from build123d import *

# Parameters (mm, degrees)
F1_DEPTH = 10
F2_R     = 4


with BuildPart() as f1:
    # F0 (on Top) → F1 (new body)
    with BuildSketch(Plane.XY):
        with BuildLine():
            Line((-14.4176203235, -8.0238534513), (-15.1564685919, -6.5216148171))
            ThreePointArc((-15.1564685919, -6.5216148171), (-14.8061090102, -7.2821106815), (-14.4176203235, -8.0238534513))
        make_face()
        with BuildLine():
            ThreePointArc((14.4176203235, -8.0238534513), (0, -16.5), (-14.4176203235, -8.0238534513))
            Line((-14.4176203235, -8.0238534513), (0, -37.3379997909))
            Line((0, -37.3379997909), (14.4176203235, -8.0238534513))
        make_face()
        with BuildLine():
            ThreePointArc((14.4176203235, -8.0238534513), (14.8061090102, -7.2821106815), (15.1564685919, -6.5216148171))
            Line((15.1564685919, -6.5216148171), (14.4176203235, -8.0238534513))
        make_face()
        with BuildLine():
            ThreePointArc((15.1564685919, -6.5216148171), (16.1606270263, -3.329284325), (16.5, 0))
            ThreePointArc((16.5, 0), (-3.329284325, 16.1606270263), (-15.1564685919, -6.5216148171))
            Line((-15.1564685919, -6.5216148171), (-14.4176203235, -8.0238534513))
            ThreePointArc((-14.4176203235, -8.0238534513), (0, -16.5), (14.4176203235, -8.0238534513))
            Line((14.4176203235, -8.0238534513), (15.1564685919, -6.5216148171))
        make_face()
    extrude(amount=F1_DEPTH)

    # F2
    f2_edges = [f1.edges().sort_by_distance(p)[0] for p in [
        (0, -37.338, 5),
    ]]
    fillet(f2_edges, radius=F2_R)


solid = f1.part
Geometry check sheet. Reference: the model listing, model coordinates, mm. Give positions to 0.01 mm unless a question says otherwise; leave off trailing zeros. Order: outer loops, then holes, each group sorted by start corner. A loop starts at its lowest first (then second) coordinate and runs counter-clockwise, first axis right, second up.
1) Cross-section at C-C (x = 7). Record the boundary of the cut face in (y, z).
Results are:
outline: (-23.11, 0) - (14.94, 0) - (14.94, 10) - (-23.11, 10) - close
2) Material ranges on probe 1 along X at (y, z) = (-6.5, 8.5); probe 2 along X at (y, z) = (5.5, 7.25); probe 3 along Y at (x, z) = (-12.5, 1.5), recorded low to high.
Results are:
probe 1: x = -15.17 to 15.17
probe 2: x = -15.56 to 15.56
probe 3: y = -11.92 to 10.77
3) Cross-section at B-B (y = -21.5). Record the boundary of the cut face in (x, z).
Results are:
outline: (-7.79, 0) - (7.79, 0) - (7.79, 10) - (-7.79, 10) - close
4) Cross-section at A-A (z = 4). Record the boundary of the cut face in (x, y), then the cut area to 3 significant figures.
Results are:
outline: (-14.42, -8.02) - (-3.59, -30.04) arc R4 ccw to (3.59, -30.04) - (14.42, -8.02) arc R16.5 ccw (long way) to start
area: 1,090 mm2
5) Gauge pin test, flat ends, axial feed: pin 1 (1 mm diameter, centred on x = 5.5, z = 8, fed in from +Y); pin 2 (1.5 mm diameter, centred on x = -6.5, z = 2, fed in from +Y); pin 3 (6 mm diameter, centred on x = 7.5, z = 3.5, fed in from -Y). Record the tip position at first contact, or that the pin passes through.
Results are:
pin 1: stops at y = 15.72
pin 2: stops at y = 15.47
pin 3: stops at y = -28.19
